The model under review builds one solid part; all positions refer to its coordinate system, in mm. A direction names the side the tool comes from. Give positions to 0.01 mm unless a question says otherwise; leave off trailing zeros. Loops run counter-clockwise (first coordinate to the right, second up) from the corner with the lowest first, then second, coordinate; pieces in that order, holes last. Notation, with made-up numbers: (89.5, 87) - (135.5, 87) arc R24 cw to (135.5, 119) - close; hole circle Ø11 at (84.5, 56.5). An arc over 180 degrees is marked (long way). Return JSON: item names as keys, results as strings. Group by question number.
from build123d import *

# Parameters (mm, degrees)
SKETCH1_W            = 20.1
SKETCH1_H            = 6
SKETCH6_R            = 2.7
CUT_EXTRUDE2_DEPTH   = 30.052022305
CUT_EXTRUDE3_DEPTH   = 2.6
M3_CLEARANCE_HOLE2_D = 3.2
CIRPATTERN1_COUNT    = 6


# Read off the part's stored shape, not the designer's step: CSK for M3 Hex Socket Countersunk Cap Screw1
with BuildPart() as part:
    # Sketch1 → Revolve1 (revolve)
    with BuildSketch(Plane.XY, mode=Mode.PRIVATE) as revolve1_sk:
        with Locations((10.05, 3)):
            Rectangle(SKETCH1_W, SKETCH1_H)
    revolve(revolve1_sk.sketch.rotate(Axis((0, 0, 0), (0, 1, 0)), 90), axis=Axis((0, 0, 0), (0, 1, 0)))

    # Sketch6 → Cut-Extrude2 (cut, through all)
    with BuildSketch(Plane(origin=(0, 6, 0), x_dir=(1, 0, 0), z_dir=(0, 1, 0))):
        with Locations(Location((0, 0, 0), (0, 0, 270))):
            Circle(SKETCH6_R)
    extrude(amount=-CUT_EXTRUDE2_DEPTH, mode=Mode.SUBTRACT)

    # Sketch9 → Cut-Extrude3 (cut)
    with BuildSketch(Plane.XZ):
        Polygon((16, 3.233161507), (13.2, 1.616580754), (13.2, -1.616580754), (16, -3.233161507), (18.8, -1.616580754), (18.8, 1.616580754), align=None)
    cut_extrude3 = extrude(amount=-CUT_EXTRUDE3_DEPTH, mode=Mode.SUBTRACT)

    # M3 Clearance Hole2 (through all)
    with Locations(Plane(origin=(0, 2.6, 0), x_dir=(-1, 0, 0), z_dir=(0, -1, 0))):
        with Locations((-16, 0)):
            m3_clearance_hole2 = Hole(M3_CLEARANCE_HOLE2_D / 2)

    # CirPattern1: Cut-Extrude3, M3 Clearance Hole2 ×6 about axis
    cirpattern1_axis = Axis((0, 0, 0), (0, 1, 0))
    add([cut_extrude3.rotate(cirpattern1_axis, i * 360 / CIRPATTERN1_COUNT) for i in range(1, CIRPATTERN1_COUNT)], mode=Mode.SUBTRACT)
    add([m3_clearance_hole2.rotate(cirpattern1_axis, i * 360 / CIRPATTERN1_COUNT) for i in range(1, CIRPATTERN1_COUNT)], mode=Mode.SUBTRACT)

    # CSK for M3 Hex Socket Countersunk Ca 2 → CSK for M3 Hex Socket Countersunk Cap Screw1 (revolve, cut)
    with BuildSketch(Plane(origin=(-13.856406461, 0, 8), x_dir=(1, 0, 0), z_dir=(0, 0, 1))):
        Polygon((0, 0), (1.8, 0), (1.8, 4.44), (3.36, 6), (0, 6), align=None)
    revolve(axis=Axis((-13.856406461, 0, 8), (0, 1, 0)), mode=Mode.SUBTRACT)

    # CSK for M3 Hex Socket Countersunk Ca 3 o → CSK for M3 Hex Socket Countersunk Ca 3 (revolve, cut)
    with BuildSketch(Plane(origin=(-13.856406461, 0, -8), x_dir=(1, 0, 0), z_dir=(0, 0, 1))):
        Polygon((0, 0), (1.8, 0), (1.8, 4.44), (3.36, 6), (0, 6), align=None)
    revolve(axis=Axis((-13.856406461, 0, -8), (0, 1, 0)), mode=Mode.SUBTRACT)

    # CSK for M3 Hex Socket Countersunk Ca 4 o → CSK for M3 Hex Socket Countersunk Ca 4 (revolve, cut)
    with BuildSketch(Plane.XY.offset(-16)):
        Polygon((0, 0), (1.8, 0), (1.8, 4.44), (3.36, 6), (0, 6), align=None)
    revolve(axis=Axis((0, 0, -16), (0, 1, 0)), mode=Mode.SUBTRACT)

    # CSK for M3 Hex Socket Countersunk Ca 5 o → CSK for M3 Hex Socket Countersunk Ca 5 (revolve, cut)
    with BuildSketch(Plane(origin=(13.856406461, 0, -8), x_dir=(1, 0, 0), z_dir=(0, 0, 1))):
        Polygon((0, 0), (1.8, 0), (1.8, 4.44), (3.36, 6), (0, 6), align=None)
    revolve(axis=Axis((13.856406461, 0, -8), (0, 1, 0)), mode=Mode.SUBTRACT)

    # CSK for M3 Hex Socket Countersunk Ca 6 o → CSK for M3 Hex Socket Countersunk Ca 6 (revolve, cut)
    with BuildSketch(Plane(origin=(13.856406461, 0, 8), x_dir=(1, 0, 0), z_dir=(0, 0, 1))):
        Polygon((0, 0), (1.8, 0), (1.8, 4.44), (3.36, 6), (0, 6), align=None)
    revolve(axis=Axis((13.856406461, 0, 8), (0, 1, 0)), mode=Mode.SUBTRACT)

    # CSK for M3 Hex Socket Countersunk Ca 7 o → CSK for M3 Hex Socket Countersunk Ca 7 (revolve, cut)
    with BuildSketch(Plane.XY.offset(16)):
        Polygon((0, 0), (1.8, 0), (1.8, 4.44), (3.36, 6), (0, 6), align=None)
    revolve(axis=Axis((0, 0, 16), (0, 1, 0)), mode=Mode.SUBTRACT)


solid = part.part
Item 1: Take a section at B-B (z = 0). State the section outline as (x, y) points.
Item 2: Tool access review of faces 1 (the face through (0.811, 3.042, 2.575)), 2 (the face through (18.8, 1, 0)): name each direction out of +Z, -Z, +X, -X, +Y, -Y from which nothing blocks a thin tool from reaching the whole face with its end or side.
Item 3: Mouldability with a two-part tool opening along X and no side actions: class faces 3 (the face through (5.2, 1, -14)), 4 (the face through (4, 0, 0)) as +X half, -X half, draft (parallel to the pull), parting line (faces both ways), or undercut.
Item 4: For L1, parallel to X at y = 2.5, z = 0; L2, parallel to X at y = 0.7, z = -8; L3, parallel to Z at x = 12.5, y = 0.7, list the stretches that pass through material, from the lowest coordinate up. Write a range as from..to.
Item 5: Take a section at A-A (x = 0). State the section outline as (y, z) points, then the cut area to 3 significant figures.
Item 6: For P1, Ø2, axis at y = 1.5, z = -14, coming from the -X side; P2, Ø3.5, axis at x = 8, z = -13.86, coming from the +Y side; P3, Ø1.3, axis at y = 1, z = 0, coming from the +X side; P4, Ø3, axis at x = -13.86, z = 8, coming from the +Y side, all flat-tipped, find the tip position at first contact; note any pin that passes through.
Item 7: Take a section at D-D (y = 5.35). State how many separate pieces and enclosed holes the cut face has, then the cut area to 3 significant figures.
Item 8: Take a section at C-C (z = 8). State the section outline as (x, y) points.
Check sheet entries:
{
 "1": {"outline": "(-20.1, 0) - (-18.8, 0) - (-18.8, 2.6) - (-17.6, 2.6) - (-17.6, 6) - (-20.1, 6) - close; (-14.4, 2.6) - (-13.2, 2.6) - (-13.2, 0) - (-2.7, 0) - (-2.7, 6) - (-14.4, 6) - close; (2.7, 0) - (13.2, 0) - (13.2, 2.6) - (14.4, 2.6) - (14.4, 6) - (2.7, 6) - close; (17.6, 2.6) - (18.8, 2.6) - (18.8, 0) - (20.1, 0) - (20.1, 6) - (17.6, 6) - close"},
 "2": {"face 1": "+Y, -Y", "face 2": "-Y"},
 "3": {"face 3": "undercut", "face 4": "draft"},
 "4": {"L1": "x = -20.1..-18.8, -13.2..-2.7, 2.7..13.2, 18.8..20.1", "L2": "x = -18.44..-15.66, -12.06..12.06, 15.66..18.44", "L3": "z = -15.74..-9.18, -6.82..6.82, 9.18..15.74"},
 "5": {"outline": "(0, -20.1) - (6, -20.1) - (6, -19.36) - (4.44, -17.8) - (0, -17.8) - close; (0, -14.2) - (4.44, -14.2) - (6, -12.64) - (6, -2.7) - (0, -2.7) - close; (0, 2.7) - (6, 2.7) - (6, 12.64) - (4.44, 14.2) - (0, 14.2) - close; (0, 17.8) - (4.44, 17.8) - (6, 19.36) - (6, 20.1) - (0, 20.1) - close", "area": "161 mm^2"},
 "6": {"P1": "stops at x = -15.33", "P2": "stops at y = 6", "P3": "stops at x = 20.1", "P4": "passes through"},
 "7": {"separate pieces": "1", "enclosed holes": "13", "area": "1,060 mm^2"},
 "8": {"outline": "(-18.44, 0) - (-15.66, 0) - (-15.66, 4.44) - (-17.22, 6) - (-18.44, 6) - close; (-12.06, 0) - (12.06, 0) - (12.06, 4.44) - (10.5, 6) - (-10.5, 6) - (-12.06, 4.44) - close; (15.66, 0) - (18.44, 0) - (18.44, 6) - (17.22, 6) - (15.66, 4.44) - close"}
}
